```python
from build123d import *

# Parameters (mm, degrees)
EXTRUDE1_DEPTH                                   = 79.502
CBORE_FOR_3_8_SOCKET_HEAD_CAP_SCREW1_D           = 10.31748
CBORE_FOR_3_8_SOCKET_HEAD_CAP_SCREW1_CBORE_D     = 16.51
CBORE_FOR_3_8_SOCKET_HEAD_CAP_SCREW1_CBORE_DEPTH = 50.165
CBORE_FOR_3_8_SOCKET_HEAD_CAP_SCREW2_D           = 10.31748
CBORE_FOR_3_8_SOCKET_HEAD_CAP_SCREW2_CBORE_D     = 16.51
CBORE_FOR_3_8_SOCKET_HEAD_CAP_SCREW2_CBORE_DEPTH = 50.165
SKETCH14_W                                       = 25.4
SKETCH14_H                                       = 12.279702398
EXTRUDE2_DEPTH                                   = 80.502
CBORE_FOR_1_2_SOCKET_HEAD_CAP_SCREW1_D           = 13.49248
CBORE_FOR_1_2_SOCKET_HEAD_CAP_SCREW1_CBORE_D     = 20.6375
CBORE_FOR_1_2_SOCKET_HEAD_CAP_SCREW1_CBORE_DEPTH = 68.58
EXTRUDE3_DEPTH                                   = 80.502
CHAMFER1_SIZE                                    = 0.762


with BuildPart() as part:
    # Sketch1 → Extrude1 (new body)
    with BuildSketch(Plane(origin=(0, 0, 0), x_dir=(1, 0, 0), z_dir=(0, 1, 0))):
        Polygon((-64.77, 36.195), (-64.77, -36.195), (64.77, -36.195), (64.77, 44.162668668), (3.17795769, 2.843029897), align=None)
    extrude(amount=EXTRUDE1_DEPTH)

    # CBORE for 3/8 Socket Head Cap Screw1 (through all)
    with Locations(Plane(origin=(-27.357474291, 0, 55.735373351), x_dir=(-0.897690082, 0, -0.440627412), z_dir=(-0.440627412, 0, 0.897690082))):
        with Locations((58.851895807, -48.26), (58.851895807, -22.86)):
            CounterBoreHole(CBORE_FOR_3_8_SOCKET_HEAD_CAP_SCREW1_D / 2, CBORE_FOR_3_8_SOCKET_HEAD_CAP_SCREW1_CBORE_D / 2, CBORE_FOR_3_8_SOCKET_HEAD_CAP_SCREW1_CBORE_DEPTH)

    # CBORE for 3/8 Socket Head Cap Screw2 (through all)
    with Locations(Plane(origin=(36.462488364, 0, 54.351857685), x_dir=(-0.830439574, 0, 0.55710871), z_dir=(0.55710871, 0, 0.830439574))):
        with Locations((-52.990978547, -25.4), (-52.990978547, -53.975)):
            CounterBoreHole(CBORE_FOR_3_8_SOCKET_HEAD_CAP_SCREW2_D / 2, CBORE_FOR_3_8_SOCKET_HEAD_CAP_SCREW2_CBORE_D / 2, CBORE_FOR_3_8_SOCKET_HEAD_CAP_SCREW2_CBORE_DEPTH)

    # Sketch14 → Extrude2 (cut, through all)
    with BuildSketch(Plane(origin=(0, 79.502, 0), x_dir=(1, 0, 0), z_dir=(0, 1, 0))):
        with Locations((1.21000637, 3.902881096)):
            Rectangle(SKETCH14_W, SKETCH14_H)
    extrude(amount=-EXTRUDE2_DEPTH, mode=Mode.SUBTRACT)

    # CBORE for 1/2 Socket Head Cap Screw1 (through all)
    with Locations(Plane.XZ):
        with Locations((-44.2976, 10.795), (42.545, 10.795)):
            CounterBoreHole(CBORE_FOR_1_2_SOCKET_HEAD_CAP_SCREW1_D / 2, CBORE_FOR_1_2_SOCKET_HEAD_CAP_SCREW1_CBORE_D / 2, CBORE_FOR_1_2_SOCKET_HEAD_CAP_SCREW1_CBORE_DEPTH)

    # Sketch17 → Extrude3 (cut, through all)
    with BuildSketch(Plane.XZ):
        Polygon((-64.77, -30.609192285), (-62.560551309, -35.110501375), (-64.77, -36.195), align=None)
        Polygon((64.77, -44.162668668), (54.288806225, -37.131254796), (64.77, -21.507736545), align=None)
    extrude(amount=-EXTRUDE3_DEPTH, mode=Mode.SUBTRACT)

    # Chamfer1
    chamfer1_edges = [part.edges().sort_by_distance(p)[0] for p in [
        (0, 79.502, 36.195),
        (59.529403112, 79.502, -29.319495671),
        (59.529403112, 0, -29.319495671),
        (64.77, 79.502, 7.343631727),
        (-37.025272469, 0, -22.576616835),
        (-37.025272469, 79.502, -22.576616835),
        (64.77, 0, 7.343631727),
        (0, 0, 36.195),
        (-64.77, 0, 2.792903858),
        (-64.77, 79.502, 2.792903858),
        (-63.665275654, 79.502, -32.85984683),
        (64.77, 39.751, 36.195),
        (-63.665275654, 0, -32.85984683),
        (-64.77, 39.751, 36.195),
        (34.099406297, 0, -23.586993546),
        (34.099406297, 79.502, -23.586993546),
    ]]
    chamfer(chamfer1_edges, length=CHAMFER1_SIZE)


solid = part.part
```
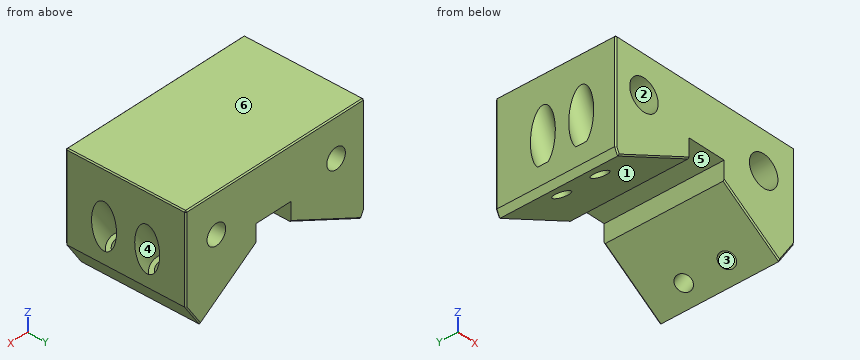
Geometry check sheet. Reference: the model listing, model coordinates, mm. Face numbers are marked on the shaded views. A direction names the side the tool comes from. Coordinates: 2 decimals unless noted, no trailing zeros. Loops run counter-clockwise (first coordinate to the right, second up) from the corner with the lowest first, then second, coordinate; pieces in that order, holes last.
Item 1: Sectioned sample at C-C, the plane x = 22.5. Record the boundary of the cut face in (y, z) (3 decimals).
Item 2: Sectioned sample at D-D, the plane z = 5.5. Count the separate pieces of the cut face and the enclosed holes in it, then the cut area to 3 significant figures.
Item 3: Sectioned sample at A-A, the plane x = -40. Record the boundary of the cut face in (y, z) (3 decimals).
Item 4: Go/stop test with flat-tipped pins: pin 1 Ø1.5 at (x, y) = (-28.5, 24.5) entering from -Z; pin 2 Ø6 at (y, z) = (46, -2.5) entering from -X; pin 3 Ø4 at (x, z) = (21.5, -17.5) entering from +Y. Record where each tip stops, or that it passes through.
Item 5: Thickness scan on line 1 (Y direction, x = 56.5, z = -10.5); line 2 (X direction, y = 31, z = 8); line 3 (X direction, y = 34, z = 16). Record the ranges inside material, lowest first.
Item 6: Access from +Z, -Z, +X, -X, +Y, -Y to the whole of each face (thin tool, end or side, straight path). Record for the marked faces 1, 2 and 3.
Item 7: Release check for a two-part mould opening along Z. For the marked faces 4, 5 and 6 record: released by +Z, released by -Z, zero draft, split by the parting line, or undercut.
Item 8: Sectioned sample at B-B, the plane y = 66.5. Record the boundary of the cut face in (x, z) (1 decimal), then the cut area to 3 significant figures.
Check result:
1. outline: (0, -14.888) - (0.762, -15.805) - (78.74, -15.805) - (79.502, -14.888) - (79.502, 35.433) - (78.74, 36.195) - (0.762, 36.195) - (0, 35.433) - close
2. separate pieces: 3
2. enclosed holes: 0
2. area: 7,390 mm2
3. outline: (0, -23.188) - (0.762, -24.037) - (78.74, -24.037) - (79.502, -23.188) - (79.502, 5.595) - (68.58, 5.595) - (68.58, 1.414) - (0, 1.414) - close; (0, 20.176) - (68.58, 20.176) - (68.58, 15.995) - (79.502, 15.995) - (79.502, 35.433) - (78.74, 36.195) - (0.762, 36.195) - (0, 35.433) - close
4. pin 1: stops at z = -18.76
4. pin 2: stops at x = -57.63
4. pin 3: stops at y = 78.78
5. line 1: y = 0 to 17.15, 33.65 to 45.72, 62.23 to 79.5
5. line 2: x = -64.77 to -54.23, -34.36 to 32.61, 52.48 to 61.87
5. line 3: x = -64.77 to -53.21, -35.39 to 33.64, 51.45 to 64.77
6. face 1: -Z, +Y, -Y
6. face 2: -Y
6. face 3: none
7. face 4: undercut
7. face 5: released by -Z
7. face 6: released by +Z
8. outline: (-64.8, -30.6) - (-62.6, -35.1) - (-11.5, -10) - (-11.5, 2.2) - (13.9, 2.2) - (13.9, -10) - (54.3, -37.1) - (64.8, -21.5) - (64.8, 35.4) - (64, 36.2) - (-64, 36.2) - (-64.8, 35.4) - close; hole circle Ø20.6 at (-44.3, 10.8); hole circle Ø20.6 at (42.5, 10.8)
8. area: 6,450 mm2
